from build123d import *

# Parameters (mm, degrees)
SKETCH1_W           = 230
SKETCH1_H           = 230
SKETCH1_R           = 2.75
SKETCH1_W_2         = 13
SKETCH1_H_2         = 49.999466707
BOSS_EXTRUDE1_DEPTH = 3.175


with BuildPart() as part:
    # Sketch1 → Boss-Extrude1 (new body)
    with BuildSketch(Plane.XY.offset(3.175)):
        Rectangle(SKETCH1_W, SKETCH1_H)
        with Locations((-26.847424973, -15.500368035)):
            Circle(SKETCH1_R, mode=Mode.SUBTRACT)
        with Locations((26.847424973, -15.500368035)):
            Circle(SKETCH1_R, mode=Mode.SUBTRACT)
        with Locations((0, 31.00073607)):
            Circle(SKETCH1_R, mode=Mode.SUBTRACT)
        with Locations((0, -47.199733354)):
            Rectangle(SKETCH1_W_2, SKETCH1_H_2, mode=Mode.SUBTRACT)
        Polygon((15.988970715, 16.736769417), (59.348272994, 41.634913462), (65.821859492, 30.361374627), (22.462557213, 5.463230583), align=None, mode=Mode.SUBTRACT)
        Polygon((-65.776572308, 30.470568229), (-59.276572308, 41.728898478), (-15.975763964, 16.729165125), (-22.475763964, 5.470834875), align=None, mode=Mode.SUBTRACT)
    extrude(amount=-BOSS_EXTRUDE1_DEPTH)


solid = part.part
Design review of the part built by this model. Coordinates are the model's own, in mm. A direction names the side the tool comes from. Coordinates: 2 decimals unless noted, no trailing zeros. Write each loop counter-clockwise with the first axis right and the second up, starting at its lowest first coordinate (ties: lowest second). Pieces come first, ordered by that corner, then holes. Notation, with made-up numbers: (46.5, 6) -> (77.5, 6) arc R25 cw to (77.5, 30) -> close; hole circle Ø6 at (54.25, -7). An arc over 180 degrees is marked (long way). Write each question's results on one line, items separated by ' | '. Start each with the question number.
(1) For line 1 along Y through (x, z) = (0, 2); line 2 along X through (y, z) = (-53.5, 2.4); line 3 along Y through (x, z) = (-6, 1.45), list the stretches that pass through material, from the lowest coordinate up. Write a range as from..to.
(2) Take a section at C-C on z = 1.8. Write out the cut boundary in (x, y).
(3) Take a section at B-B on x = 0. Write out the cut boundary in (y, z) (3 decimals), and give its area (3 significant figures).
(4) The part is to be moulded in two halves that separate along X. For faces 3 (the face through (-19.18, 11.18, 1.61)), 4 (the face through (-2, 2, 0)), say which applies: pulls with the +X half, pulls with the -X half, needs draft (parallel to the pull), parting line crosses it, or undercut.
(5) Tool access review of faces 1 (the face through (37.365, 29.012, 1.61)), 2 (the face through (-2, 2, 3.175)): name each direction out of +Z, -Z, +X, -X, +Y, -Y from which nothing blocks a thin tool from reaching the whole face with its end or side.
(6) Take a section at A-A on y = -56.5. Write out the cut boundary in (x, z) (3 decimals), and give its area (3 significant figures).
Results found:
1) line 1: y = -115..-72.2, -22.2..28.25, 33.75..115 | line 2: x = -115..-6.5, 6.5..115 | line 3: y = -115..-72.2, -22.2..115
2) outline: (-115, -115) -> (115, -115) -> (115, 115) -> (-115, 115) -> close; hole (-65.78, 30.47) -> (-22.48, 5.47) -> (-15.98, 16.73) -> (-59.28, 41.73) -> close; hole circle Ø5.5 at (-26.85, -15.5); hole (-6.5, -72.2) -> (6.5, -72.2) -> (6.5, -22.2) -> (-6.5, -22.2) -> close; hole circle Ø5.5 at (0, 31); hole (15.99, 16.74) -> (22.46, 5.46) -> (65.82, 30.36) -> (59.35, 41.63) -> close; hole circle Ø5.5 at (26.85, -15.5)
3) outline: (-115, 0) -> (-72.199, 0) -> (-72.199, 3.175) -> (-115, 3.175) -> close; (-22.2, 0) -> (28.251, 0) -> (28.251, 3.175) -> (-22.2, 3.175) -> close; (33.751, 0) -> (115, 0) -> (115, 3.175) -> (33.751, 3.175) -> close | area: 554 mm2
4) face 3: undercut | face 4: needs draft
5) face 1: +Z, -Z | face 2: +Z, +X, -X, +Y, -Y
6) outline: (-115, 0) -> (-6.5, 0) -> (-6.5, 3.175) -> (-115, 3.175) -> close; (6.5, 0) -> (115, 0) -> (115, 3.175) -> (6.5, 3.175) -> close | area: 689 mm2
